```python
from build123d import *

# Parameters (mm, degrees)
SKETCH_1_R      = 1.1303
EXTRUDE_1_DEPTH = 1.588


with BuildPart() as part:
    # 草图1 → 凸台-拉伸1 (new body)
    with BuildSketch(Plane(origin=(-0.79375, 0, 0), x_dir=(0, -1, 0), z_dir=(-1, 0, 0))):
        with BuildLine():
            Line((40.795, -5.078289511), (40.795, 3))
            ThreePointArc((40.795, 3), (40.209213562, 4.414213562), (38.795, 5))
            Line((38.795, 5), (12.795, 5))
            ThreePointArc((12.795, 5), (11.380786438, 4.414213562), (10.795, 3))
            Line((10.795, 3), (10.795, -13))
            ThreePointArc((10.795, -13), (11.380786438, -14.414213562), (12.795, -15))
            Line((12.795, -15), (33.193504795, -15))
            ThreePointArc((33.193504795, -15), (34.112906481, -14.776147668), (34.826497957, -14.154700538))
            Line((34.826497957, -14.154700538), (40.427993162, -6.232990049))
            ThreePointArc((40.427993162, -6.232990049), (40.701041228, -5.684100404), (40.795, -5.078289511))
        make_face()
        with Locations((18.295, 0)):
            Circle(SKETCH_1_R, mode=Mode.SUBTRACT)
        with Locations((13.295, 0)):
            Circle(SKETCH_1_R, mode=Mode.SUBTRACT)
    extrude(amount=-EXTRUDE_1_DEPTH)


solid = part.part
```
Geometry: final body of the model. Coordinates: model frame, mm. Round coordinates to 2 decimals unless told otherwise and drop trailing zeros. Order: outer loops, then holes, each group sorted by start corner. A loop starts at its lowest first (then second) coordinate and runs counter-clockwise, first axis right, second up. Notation, with made-up numbers: (49, 25.5) -> (88, 25.5) arc R28 cw to (88, 53.5) -> close; hole circle Ø3 at (-9.75, -3). An arc over 180 degrees is marked (long way). Use one line per item in the form item = value.
(1) Section C-C on y = -34.5. Return loops of the section in (x, z).
Results list:
outline = (-0.79, -14.51) -> (0.79, -14.51) -> (0.79, 5) -> (-0.79, 5) -> close
(2) Draft query along Y for faces 1 (the face through (-0.011, -34.101, -14.782)), 2 (the face through (0.794, -26, -5)), 3 (the face through (-0.011, -11.396, 4.43)), 4 (the face through (-0.01, -19.34, -0.43)). Return one class per face: pulls with the +Y half, pulls with the -Y half, needs draft (parallel to the pull), parting line crosses it, or undercut.
Results list:
face_1 = pulls with the -Y half
face_2 = needs draft
face_3 = pulls with the +Y half
face_4 = undercut
(3) First-contact query: pin 1 Ø1.4 at (y, z) = (-18.295, 0) entering from +X. Flat tip, straight axial feed; report the tip coordinate or a pass-through.
Results list:
pin_1 = through
(4) Ray query, probe 1 along Y at (x, z) = (0.1, 1) (3 decimals); probe 2 along Z at (x, y) = (-0.6, -19); probe 3 along Z at (x, y) = (0.65, -36.5). Return the intervals inside material, ascending. Write a range as [from, to].
Results list:
probe_1 = [-40.795, -18.822], [-17.768, -13.822], [-12.768, -10.795]
probe_2 = [-15, -0.88], [0.88, 5]
probe_3 = [-11.79, 5]
(5) Section A-A on z = 0. Return loops of the section in (x, y) (3 decimals).
Results list:
outline = (-0.794, -40.795) -> (0.794, -40.795) -> (0.794, -19.425) -> (-0.794, -19.425) -> close; (-0.794, -17.165) -> (0.794, -17.165) -> (0.794, -14.425) -> (-0.794, -14.425) -> close; (-0.794, -12.165) -> (0.794, -12.165) -> (0.794, -10.795) -> (-0.794, -10.795) -> close
(6) Section B-B on x = 0.05. Return loops of the section in (y, z) (1 decimal), and give its area (3 significant figures).
Results list:
outline = (-40.8, -5.1) arc R2 ccw to (-40.4, -6.2) -> (-34.8, -14.2) arc R2 ccw to (-33.2, -15) -> (-12.8, -15) arc R2 ccw to (-10.8, -13) -> (-10.8, 3) arc R2 ccw to (-12.8, 5) -> (-38.8, 5) arc R2 ccw to (-40.8, 3) -> close; hole circle Ø2.3 at (-18.3, 0); hole circle Ø2.3 at (-13.3, 0)
area = 559 mm^2
